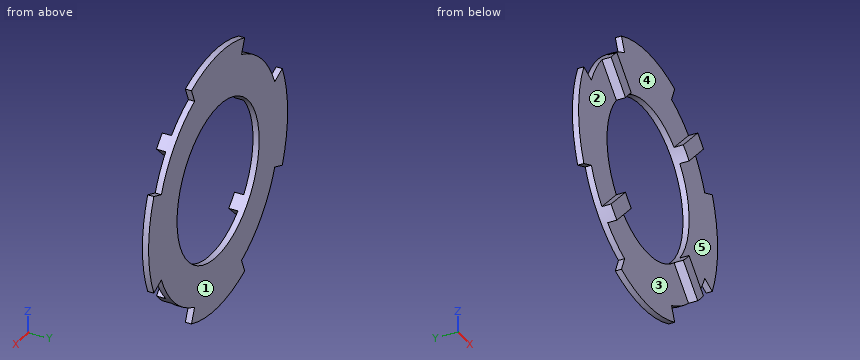
Autodesk Inventor part; units mm, degrees
ref_plane "YZ Plane" through (0, 0, 0) normal (1, 0, 0) x (0, 1, 0)
ref_plane "XZ Plane" through (0, 0, 0) normal (0, 1, 0) x (-1, 0, 0)
ref_plane "XY Plane" through (0, 0, 0) normal (0, 0, 1) x (1, 0, 0)
sketch "Sketch1" plane through (0, 0, 0) normal (0, 1, 0) x (-1, 0, 0)
  circle A0 centre (0, 0) radius 42.75
  circle A1 centre (0, 0) radius 25.25
  dimension "d0" = 85.5
  dimension "d1" = 50.5
extrude "Extrusion1" add sketch "Sketch1" along normal blind 2
sketch "Sketch2" plane through (0, 2, 0) normal (0, 1, 0) x (1, 0, 0)
  circle A0 centre (0, 0) radius 25.25
  circle A1 centre (0, 0) radius 42.75
  line L0 (0, 0) -> (26.6933, 26.6933)
  arc A2 (39.4959, 16.3597) -> (30.2288, 30.2288) centre (0, 0) ccw
  line L1 (0, 0) -> (39.4959, 16.3597) construction
  line L2 (0, 0) -> (26.6933, 26.6933) construction
  arc A3 (30.2288, 30.2288) -> (16.3597, 39.4959) centre (0, 0) ccw
  line L3 (0, 0) -> (30.2288, 30.2288) construction
  line L4 (0, 0) -> (17.5537, 7.271) construction
  line L5 (0, 0) -> (17.8544, 17.8544) construction
  line L6 (0, 0) -> (9.6628, 23.328) construction
  line L7 (0, 0) -> (17.8544, 17.8544) construction
  line L8 (16.3597, 39.4959) -> (14.4463, 34.8765)
  line L9 (34.8765, 14.4463) -> (39.4959, 16.3597)
  arc A4 (34.8765, 14.4463) -> (14.4463, 34.8765) centre (0, 0) ccw
  line L10 (16.3597, 39.4959) -> (14.4463, 34.8765)
  line L11 (39.4959, 16.3597) -> (34.8765, 14.4463)
  line L12 (0, 0) -> (9.6628, 23.328) construction
  line L13 (14.4463, 34.8765) -> (16.3597, 39.4959) construction
  line L14 (-39.4959, 16.3597) -> (-34.8765, 14.4463)
  arc A5 (-30.2288, 30.2288) -> (-39.4959, 16.3597) centre (0, 0) ccw
  arc A6 (-16.3597, 39.4959) -> (-30.2288, 30.2288) centre (0, 0) ccw
  line L15 (-14.4463, 34.8765) -> (-16.3597, 39.4959)
  arc A7 (-14.4463, 34.8765) -> (-34.8765, 14.4463) centre (0, 0) ccw
  line L16 (-16.3597, -39.4959) -> (-14.4463, -34.8765)
  arc A8 (-30.2288, -30.2288) -> (-16.3597, -39.4959) centre (0, 0) ccw
  arc A9 (-39.4959, -16.3597) -> (-30.2288, -30.2288) centre (0, 0) ccw
  line L17 (-34.8765, -14.4463) -> (-39.4959, -16.3597)
  arc A10 (-34.8765, -14.4463) -> (-14.4463, -34.8765) centre (0, 0) ccw
  line L18 (39.4959, -16.3597) -> (34.8765, -14.4463)
  arc A11 (30.2288, -30.2288) -> (39.4959, -16.3597) centre (0, 0) ccw
  arc A12 (16.3597, -39.4959) -> (30.2288, -30.2288) centre (0, 0) ccw
  line L19 (14.4463, -34.8765) -> (16.3597, -39.4959)
  arc A13 (14.4463, -34.8765) -> (34.8765, -14.4463) centre (0, 0) ccw
  point P0 (-26.6933, 26.6933)
  point P1 (-26.6933, -26.6933)
  point P2 (26.6933, -26.6933)
  dimension "d4" = 22.5
  dimension "d8" = 75.5
  dimension "d11" = 360
extrude "Extrusion2" cut sketch "Sketch2" against normal through all contours A4 L8 A1 L9 | L15 A7 L14 A1 | A1 L19 A13 L18 | L17 A10 L16 A1
sketch "Sketch5" plane through (0, 0, 0) normal (0, -1, 0) x (1, 0, 0)
  line L0 (-16.3597, 39.4959) -> (-14.4463, 34.8765)
  line L1 (-34.8765, 14.4463) -> (-39.4959, 16.3597)
  arc A0 (-39.4959, 16.3597) -> (-39.4959, -16.3597) centre (0, 0) ccw
  line L2 (-39.4959, -16.3597) -> (-34.8765, -14.4463)
  line L3 (-14.4463, -34.8765) -> (-16.3597, -39.4959)
  arc A1 (-16.3597, -39.4959) -> (16.3597, -39.4959) centre (0, 0) ccw
  line L4 (16.3597, -39.4959) -> (14.4463, -34.8765)
  line L5 (34.8765, -14.4463) -> (39.4959, -16.3597)
  arc A2 (39.4959, -16.3597) -> (39.4959, 16.3597) centre (0, 0) ccw
  line L6 (39.4959, 16.3597) -> (34.8765, 14.4463)
  line L7 (14.4463, 34.8765) -> (16.3597, 39.4959)
  arc A3 (16.3597, 39.4959) -> (-16.3597, 39.4959) centre (0, 0) ccw
  circle A4 centre (0, 0) radius 25.25
  line L8 (0, 0) -> (-17.8544, -17.8544)
  line L9 (0, 0) -> (-5.6762, 0)
  line L10 (-19.8816, -22.7984) -> (-16.3892, -19.2083)
  line L11 (-22.8427, -19.8307) -> (-19.2083, -16.3892)
  arc A5 (-19.2083, -16.3892) -> (-16.3892, -19.2083) centre (0, 0) ccw
  arc A6 (-22.8427, -19.8307) -> (-19.8816, -22.7984) centre (0, 0) ccw
  line L12 (22.7984, -19.8816) -> (19.2083, -16.3892)
  line L13 (19.8307, -22.8427) -> (16.3892, -19.2083)
  arc A7 (16.3892, -19.2083) -> (19.2083, -16.3892) centre (0, 0) ccw
  arc A8 (19.8307, -22.8427) -> (22.7984, -19.8816) centre (0, 0) ccw
  line L14 (19.8816, 22.7984) -> (16.3892, 19.2083)
  line L15 (22.8427, 19.8307) -> (19.2083, 16.3892)
  arc A9 (19.2083, 16.3892) -> (16.3892, 19.2083) centre (0, 0) ccw
  arc A10 (22.8427, 19.8307) -> (19.8816, 22.7984) centre (0, 0) ccw
  line L16 (-22.7984, 19.8816) -> (-19.2083, 16.3892)
  line L17 (-19.8307, 22.8427) -> (-16.3892, 19.2083)
  arc A11 (-16.3892, 19.2083) -> (-19.2083, 16.3892) centre (0, 0) ccw
  arc A12 (-19.8307, 22.8427) -> (-22.7984, 19.8816) centre (0, 0) ccw
  arc A13 (-14.4463, 34.8765) -> (-34.8765, 14.4463) centre (0, 0) ccw
  arc A14 (-34.8765, -14.4463) -> (-14.4463, -34.8765) centre (0, 0) ccw
  arc A15 (14.4463, -34.8765) -> (34.8765, -14.4463) centre (0, 0) ccw
  arc A16 (34.8765, 14.4463) -> (14.4463, 34.8765) centre (0, 0) ccw
  point P0 (17.8544, -17.8544)
  point P1 (17.8544, 17.8544)
  point P2 (-17.8544, 17.8544)
  dimension "d31" = 45
  dimension "d35" = 360
extrude "Extrusion4" [suppressed]
sketch "Sketch6" plane through (0, 0, 0) normal (0, -1, 0) x (1, 0, 0)
  line L0 (-16.3597, 39.4959) -> (-14.4463, 34.8765)
  arc A0 (-14.4463, 34.8765) -> (-34.8765, 14.4463) centre (0, 0) ccw
  line L1 (-34.8765, 14.4463) -> (-39.4959, 16.3597)
  arc A1 (-39.4959, 16.3597) -> (-39.4959, -16.3597) centre (0, 0) ccw
  line L2 (-39.4959, -16.3597) -> (-34.8765, -14.4463)
  arc A2 (-34.8765, -14.4463) -> (-14.4463, -34.8765) centre (0, 0) ccw
  line L3 (-14.4463, -34.8765) -> (-16.3597, -39.4959)
  arc A3 (-16.3597, -39.4959) -> (16.3597, -39.4959) centre (0, 0) ccw
  line L4 (16.3597, -39.4959) -> (14.4463, -34.8765)
  arc A4 (14.4463, -34.8765) -> (34.8765, -14.4463) centre (0, 0) ccw
  line L5 (34.8765, -14.4463) -> (39.4959, -16.3597)
  arc A5 (39.4959, -16.3597) -> (39.4959, 16.3597) centre (0, 0) ccw
  line L6 (39.4959, 16.3597) -> (34.8765, 14.4463)
  arc A6 (34.8765, 14.4463) -> (14.4463, 34.8765) centre (0, 0) ccw
  line L7 (14.4463, 34.8765) -> (16.3597, 39.4959)
  arc A7 (16.3597, 39.4959) -> (-16.3597, 39.4959) centre (0, 0) ccw
  circle A8 centre (0, 0) radius 25.25
  line L8 (0, 0) -> (26.6933, 26.6933)
  line L9 (15.999, 19.5345) -> (19.5345, 15.999)
  arc A9 (19.5345, 15.999) -> (15.999, 19.5345) centre (0, 0) ccw
  line L10 (19.5345, 15.999) -> (28.4024, 24.8669)
  line L11 (15.999, 19.5345) -> (24.8669, 28.4024)
  arc A10 (28.4024, 24.8669) -> (24.8669, 28.4024) centre (0, 0) ccw
  line L12 (-19.5345, 15.999) -> (-15.999, 19.5345)
  arc A11 (-15.999, 19.5345) -> (-19.5345, 15.999) centre (0, 0) ccw
  line L13 (-15.999, 19.5345) -> (-24.8669, 28.4024)
  line L14 (-19.5345, 15.999) -> (-28.4024, 24.8669)
  arc A12 (-24.8669, 28.4024) -> (-28.4024, 24.8669) centre (0, 0) ccw
  line L15 (-15.999, -19.5345) -> (-19.5345, -15.999)
  arc A13 (-19.5345, -15.999) -> (-15.999, -19.5345) centre (0, 0) ccw
  line L16 (-19.5345, -15.999) -> (-28.4024, -24.8669)
  line L17 (-15.999, -19.5345) -> (-24.8669, -28.4024)
  arc A14 (-28.4024, -24.8669) -> (-24.8669, -28.4024) centre (0, 0) ccw
  line L18 (19.5345, -15.999) -> (15.999, -19.5345)
  arc A15 (15.999, -19.5345) -> (19.5345, -15.999) centre (0, 0) ccw
  line L19 (15.999, -19.5345) -> (24.8669, -28.4024)
  line L20 (19.5345, -15.999) -> (28.4024, -24.8669)
  arc A16 (24.8669, -28.4024) -> (28.4024, -24.8669) centre (0, 0) ccw
  point P0 (-26.6933, 26.6933)
  point P1 (-26.6933, -26.6933)
  point P2 (26.6933, -26.6933)
  dimension "d39" = 5
  dimension "d40" = 2.5
  dimension "d43" = 360
extrude "Extrusion5" add sketch "Sketch6" along normal blind 3 contours L13 A8 L14 A0 | A6 L8 A8 L11 | A6 L10 A8 L8 | A8 L17 A2 L16 | A8 L20 A4 L19
equation "\"d40\" = 0.5 * d39"
properties part number "Dome Clip"
Here's how the part is built. I have some questions about the finished solid (model axes, mm). Face numbers are marked on the shaded views. A direction names the side the tool comes from. Coordinates: 2 decimals unless noted, no trailing zeros. Loops run counter-clockwise (first coordinate to the right, second up) from the corner with the lowest first, then second, coordinate; pieces in that order, holes last. Notation, with made-up numbers: (59, -17.5) - (94, -17.5) arc R24 ccw to (94, -2.5) - close; hole circle Ø10 at (84.25, 11.5). An arc over 180 degrees is marked (long way). Return JSON: item names as keys, results as strings. Group by question number.
Item 1: We'd pull the mould along Z, two halves only. Please class the marked faces 1 and 2: +Z half, -Z half, draft (parallel to the pull), parting line (faces both ways), or undercut.
Item 2: Will these pins go through, and if not, where does the flat tip stop? P1, Ø5, axis at x = 28, z = 25.5, coming from the -Y side; P2, Ø7, axis at x = 31.5, z = 7.5, coming from the -Y side; P3, Ø3, axis at y = -0.5, z = 2, coming from the +X side; P4, Ø3, axis at y = 1.5, z = 25.5, coming from the +X side.
Item 3: If we section it at A-A on x = 0: Write out the boundary of the cut face in (y, z), and give its area (3 significant figures).
Item 4: I need wall thicknesses on line 1 (Y direction, x = -17, z = 25); line 2 (X direction, y = 1.65, z = 1); line 3 (Z direction, x = 3.5, y = 0.95). Which ranges of each line are inside material? Lowest first, please. Write a range as from..to.
Item 5: If we section it at B-B on z = 0: Write out the boundary of the cut face in (x, y).
Item 6: On a 3-axis mill with a long thin cutter (end or side, diameter ignored), from which of +Z, -Z, +X, -X, +Y, -Y can I reach the whole of each face in a straight line? I mean the marked faces 3, 4 and 5. Say none if no direction works.
Calculated:
{
 "1": {"face 1": "draft", "face 2": "undercut"},
 "2": {"P1": "stops at y = -3", "P2": "stops at y = 0", "P3": "stops at x = 42.75", "P4": "stops at x = 29.14"},
 "3": {"outline": "(0, -42.75) - (2, -42.75) - (2, -25.25) - (0, -25.25) - close; (0, 25.25) - (2, 25.25) - (2, 42.75) - (0, 42.75) - close", "area": "70.0 mm^2"},
 "4": {"line 1": "y = 0..2", "line 2": "x = -42.74..-25.23, 25.23..42.74", "line 3": "z = -42.61..-25.01, 25.01..42.61"},
 "5": {"outline": "(-42.75, 0) - (-25.25, 0) - (-25.25, 2) - (-42.75, 2) - close; (25.25, 0) - (42.75, 0) - (42.75, 2) - (25.25, 2) - close"},
 "6": {"face 3": "-Z, -Y", "face 4": "+Z, -Y", "face 5": "+X, -Y"}
}
